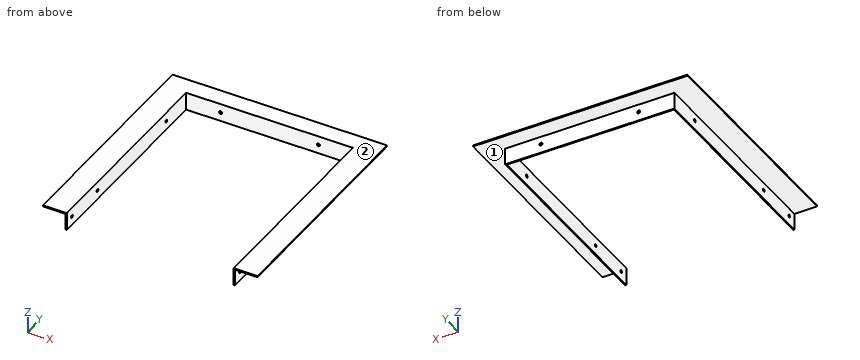
from build123d import *

# Parameters (mm, degrees)
F1_DEPTH = 38.1
F2_T     = -2.54
F3_R     = 3.175
F4_DEPTH = 408.941
F5_R     = 3.175
F6_DEPTH = 447.041


with BuildPart() as f1:
    # F0 (on Top) → F1 (new body)
    with BuildSketch(Plane.XY):
        Polygon((-177.8, -241.3), (-177.8, 203.2), (177.8, 203.2), (177.8, -241.3), (228.6, -241.3), (228.6, 241.3), (-228.6, 241.3), (-228.6, -241.3), align=None)
    extrude(amount=F1_DEPTH)

    # F2
    f2_openings = [f1.faces().sort_by_distance(p)[0] for p in [
        (-184.447816, -19.05, 0),
        (-228.6, 0, 19.05),
        (0, 241.3, 19.05),
        (228.6, 0, 19.05),
        (203.2, -241.3, 19.05),
        (-203.2, -241.3, 19.05),
    ]]
    offset(amount=F2_T, openings=f2_openings, kind=Kind.INTERSECTION)

    # F3 (on face) → F4 (cut, through all)
    with BuildSketch(Plane.YZ.offset(180.34)):
        with Locations((-222.25, 19.05)):
            Circle(F3_R)
        with Locations((-127, 19.05)):
            Circle(F3_R)
        with Locations((129.54, 19.05)):
            Circle(F3_R)
    extrude(amount=-F4_DEPTH, mode=Mode.SUBTRACT)

    # F5 (on face) → F6 (cut, through all)
    with BuildSketch(Plane(origin=(0, 205.74, 0), x_dir=(-1, 0, 0), z_dir=(0, 1, 0))):
        with Locations((-104.14, 19.05)):
            Circle(F5_R)
        with Locations((104.14, 19.05)):
            Circle(F5_R)
    extrude(amount=-F6_DEPTH, mode=Mode.SUBTRACT)


solid = f1.part
Model file for the job. Use its own axes, mm. Face numbers are marked on the shaded views. A direction names the side the tool comes from. Round coordinates to 2 decimals unless told otherwise and drop trailing zeros. Loops run counter-clockwise (first coordinate to the right, second up) from the corner with the lowest first, then second, coordinate; pieces in that order, holes last. Notation, with made-up numbers: (10, 67) -> (34, 67) arc R20 cw to (34, 98) -> close; hole circle Ø2 at (60, 66.5). An arc over 180 degrees is marked (long way). Answer as CSV lines item,"result". Start each with the question number.
1) Slice it at C-C (x = -200). List the corners of the cut face in (y, z).
2) Probe line 1 along Z through (x, y) = (-104.14, 205.15) (3 decimals); line 2 along X through (y, z) = (109.5, 15.5); line 3 along X through (y, z) = (-37, 36.5). List the from-to ranges inside material, lowest first.
3) Slice it at A-A (y = -13). List the corners of the cut face in (x, z), plus the area to 3 significant figures.
4) Tool access for the marked faces 1 and 2: list every direction of +Z, -Z, +X, -X, +Y, -Y with a clear straight run to the whole face (end or side of a thin tool).
5) Pin check, flat tips, straight feed: P1, Ø10.5, axis at y = -58, z = 11.5, coming from the +X side; P2, Ø5, axis at y = -69, z = 30, coming from the -X side; P3, Ø4, axis at y = 129.54, z = 19.05, coming from the -X side; P4, Ø8, axis at x = 109, z = 16.5, coming from the -Y side. Stop position of each tip, or through.
6) Slice it at B-B (x = -59). List the corners of the cut face in (y, z).
Filled in:
1,outline,"(-241.3, 35.56) -> (241.3, 35.56) -> (241.3, 38.1) -> (-241.3, 38.1) -> close"
2,line 1,"z = 0 to 15.875, 22.225 to 38.1"
2,line 2,"x = -180.34 to -177.8, 177.8 to 180.34"
2,line 3,"x = -228.6 to -177.8, 177.8 to 228.6"
3,outline,"(-228.6, 35.56) -> (-180.34, 35.56) -> (-180.34, 0) -> (-177.8, 0) -> (-177.8, 38.1) -> (-228.6, 38.1) -> close; (177.8, 0) -> (180.34, 0) -> (180.34, 35.56) -> (228.6, 35.56) -> (228.6, 38.1) -> (177.8, 38.1) -> close"
3,area,"439 mm2"
4,face 1,"-Z, +Y"
4,face 2,"+Z, +X, -X, +Y, -Y"
5,P1,"stops at x = 180.34"
5,P2,"stops at x = -180.34"
5,P3,"passes through"
5,P4,"stops at y = 203.2"
6,outline,"(203.2, 0) -> (205.74, 0) -> (205.74, 35.56) -> (241.3, 35.56) -> (241.3, 38.1) -> (203.2, 38.1) -> close"
